```python
from build123d import *

# Parameters (mm, degrees)
SKETCH1_W        = 19.05
SKETCH1_H        = 25.4
MAIN_BLOCK_DEPTH = 6.35
SKETCH2_W        = 6.35
SKETCH2_H        = 19.05
U_CUT_DEPTH      = 12.7
SKETCH3_R        = 1.25603
BOLT_HOLES_DEPTH = 12.7


with BuildPart() as part:
    # Sketch1 → Main block (new body)
    with BuildSketch(Plane.XY):
        with Locations((9.525, 12.7)):
            Rectangle(SKETCH1_W, SKETCH1_H)
    extrude(amount=MAIN_BLOCK_DEPTH)

    # Sketch2 → U-cut (cut)
    with BuildSketch(Plane.XY.offset(6.35)):
        with Locations((9.525, 15.875)):
            Rectangle(SKETCH2_W, SKETCH2_H)
    extrude(amount=-U_CUT_DEPTH, mode=Mode.SUBTRACT)

    # Sketch3 → Bolt holes (cut)
    with BuildSketch(Plane.XY.offset(6.35)):
        with Locations((3.175, 3.175)):
            Circle(SKETCH3_R)
        with Locations((15.875, 3.175)):
            Circle(SKETCH3_R)
    extrude(amount=-BOLT_HOLES_DEPTH, mode=Mode.SUBTRACT)


solid = part.part
```
Check sheet for the modelled part. Datum: model origin and axes. Units: mm. A direction names the side the tool comes from. Give positions to 0.01 mm unless a question says otherwise; leave off trailing zeros. Order: outer loops, then holes, each group sorted by start corner. A loop starts at its lowest first (then second) coordinate and runs counter-clockwise, first axis right, second up. Notation, with made-up numbers: M 56.5,-13.5 L 113.5,-13.5 A12 cw 113.5,-4.5 Z; hole C -20.5,60.5 d11. An arc over 180 degrees is marked long. Answer in a Markdown table with one row per item.
1) Cross-section at D-D, the plane x = 9.75. Enter the section's corners in (y, z), plus the area to 3 significant figures.
Filled sheet:
| item | result |
|---|---|
| outline | M 0,0 L 6.35,0 L 6.35,6.35 L 0,6.35 Z |
| area | 40.3 mm2 |
2) Cross-section at A-A, the plane y = 17. Enter the section's corners in (x, z).
Filled sheet:
| item | result |
|---|---|
| outline | M 0,0 L 6.35,0 L 6.35,6.35 L 0,6.35 Z; M 12.7,0 L 19.05,0 L 19.05,6.35 L 12.7,6.35 Z |
3) Release check for a two-part mould opening along X. For faces 1 (the flat face through (19.05, 13, 3)), 2 (the flat face through (0, 13, 3)), 3 (the cylindrical face through (3.75, 2.06, 3.22)), 4 (the flat face through (16, 25.4, 3)) record: +X half, -X half, draft (parallel to the pull), parting line (faces both ways), or undercut.
Filled sheet:
| item | result |
|---|---|
| face 1 | +X half |
| face 2 | -X half |
| face 3 | undercut |
| face 4 | draft |
4) Cross-section at C-C, the plane z = 2. Enter the section's corners in (x, y) (3 decimals), plus the area to 3 significant figures.
Filled sheet:
| item | result |
|---|---|
| outline | M 0,0 L 19.05,0 L 19.05,25.4 L 12.7,25.4 L 12.7,6.35 L 6.35,6.35 L 6.35,25.4 L 0,25.4 Z; hole C 3.175,3.175 d2.512; hole C 15.875,3.175 d2.512 |
| area | 353 mm2 |
5) Access from +Z, -Z, +X, -X, +Y, -Y to the whole of each face (thin tool, end or side, straight path). Record for faces 5 (the flat face through (9, 0, 3)), 6 (the flat face through (12.7, 16, 3)).
Filled sheet:
| item | result |
|---|---|
| face 5 | +Z, -Z, +X, -X, -Y |
| face 6 | +Z, -Z, +Y |
6) Thickness scan on L1, parallel to X at y = 10.75, z = 6; L2, parallel to X at y = 2.75, z = 1.25; L3, parallel to Y at x = 7.25, z = 4.75. Record the ranges inside material, lowest first. Write a range as [from, to].
Filled sheet:
| item | result |
|---|---|
| L1 | x = [0, 6.35], [12.7, 19.05] |
| L2 | x = [0, 1.99], [4.36, 14.69], [17.06, 19.05] |
| L3 | y = [0, 6.35] |
7) Cross-section at B-B, the plane x = 16.5. Enter the section's corners in (y, z), plus the area to 3 significant figures.
Filled sheet:
| item | result |
|---|---|
| outline | M 0,0 L 2.09,0 L 2.09,6.35 L 0,6.35 Z; M 4.26,0 L 25.4,0 L 25.4,6.35 L 4.26,6.35 Z |
| area | 147 mm2 |
